```python
from build123d import *

# Parameters (mm, degrees)
SKETCH1_R           = 5.6
BOSS_EXTRUDE1_DEPTH = 3
SKETCH2_R           = 8.5
SKETCH2_R_2         = 5.6
BOSS_EXTRUDE2_DEPTH = 6
SKETCH3_R           = 8.5
BOSS_EXTRUDE3_DEPTH = 6
SKETCH4_R           = 1.6
CUT_EXTRUDE1_DEPTH  = 80.186488747
SKETCH5_R           = 3.3
CUT_EXTRUDE2_DEPTH  = 1.5
BOSS_EXTRUDE4_START = 6
SKETCH6_R           = 3.25
SKETCH6_R_2         = 1.6
BOSS_EXTRUDE4_DEPTH = 0.5


with BuildPart() as part:
    # Sketch1 → Boss-Extrude1 (new body)
    with BuildSketch(Plane.XY):
        with BuildLine():
            Line((6.873863542, 5), (63.126136458, 5))
            ThreePointArc((63.126136458, 5), (78.5, 0), (63.126136458, -5))
            Line((63.126136458, -5), (6.873863542, -5))
            ThreePointArc((6.873863542, -5), (-8.5, 0), (6.873863542, 5))
        make_face()
        Circle(SKETCH1_R, mode=Mode.SUBTRACT)
    extrude(amount=BOSS_EXTRUDE1_DEPTH)

    # Sketch2 → Boss-Extrude2 (add)
    with BuildSketch(Plane.XY):
        with Locations(Location((0, 0, 0), (0, 0, 323.968120928))):
            Circle(SKETCH2_R)
        Circle(SKETCH2_R_2, mode=Mode.SUBTRACT)
    extrude(amount=BOSS_EXTRUDE2_DEPTH)

    # Sketch3 → Boss-Extrude3 (add)
    with BuildSketch(Plane.XY):
        with Locations(Location((70, 0, 0), (0, 0, 216.031879072))):
            Circle(SKETCH3_R)
    extrude(amount=BOSS_EXTRUDE3_DEPTH)

    # Sketch4 → Cut-Extrude1 (cut, through all)
    with BuildSketch(Plane.XY):
        with Locations((70, 0)):
            Circle(SKETCH4_R)
    extrude(amount=CUT_EXTRUDE1_DEPTH, mode=Mode.SUBTRACT)

    # Sketch5 → Cut-Extrude2 (cut)
    with BuildSketch(Plane.XY):
        with Locations((70, 0)):
            Circle(SKETCH5_R)
    extrude(amount=CUT_EXTRUDE2_DEPTH, mode=Mode.SUBTRACT)

    # Sketch6 → Boss-Extrude4 (add)
    with BuildSketch(Plane.XY.offset(BOSS_EXTRUDE4_START)):
        with Locations((70, 0)):
            Circle(SKETCH6_R)
        with Locations((70, 0)):
            Circle(SKETCH6_R_2, mode=Mode.SUBTRACT)
    extrude(amount=BOSS_EXTRUDE4_DEPTH)


solid = part.part
```
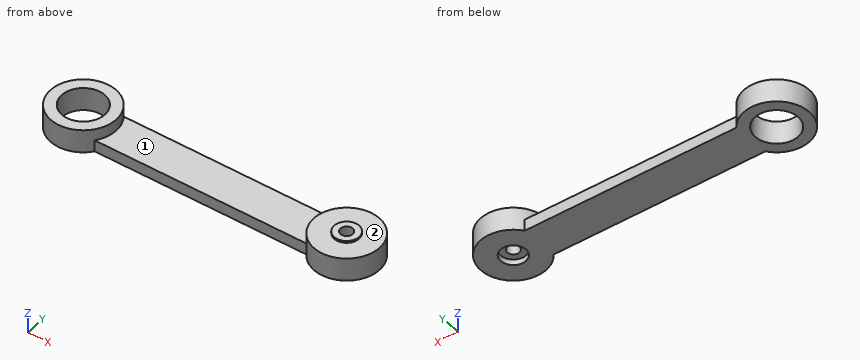
CAD build for the part. Positions are in the model's coordinates, mm. Face numbers are marked on the shaded views. Give positions to 0.01 mm unless a question says otherwise; leave off trailing zeros. Order: outer loops, then holes, each group sorted by start corner. A loop starts at its lowest first (then second) coordinate and runs counter-clockwise, first axis right, second up. Notation, with made-up numbers: M 58.25,-7 L 72.25,-7 A27 cw 72.25,30 Z; hole C 50,-7 d4. An arc over 180 degrees is marked long. Put each result on its own line as item: value. Start each with the question number.
(1) Mould opens along X. For the marked faces 1 and 2 say: +X half, -X half, draft (parallel to the pull), parting line (faces both ways), or undercut.
(2) Saw through at B-B, the plane y = 0. Write the cut outline in (x, z), then the cut area to 3 significant figures.
(3) Saw through at D-D, the plane x = 0. Write the cut outline in (y, z).
(4) Drill centre lines: line 1 along Y through (x, z) = (70, 1.15); line 2 along Y through (x, z) = (0, 2.6); line 3 along X through (y, z) = (-1.75, 3.75). Where is each one in solid material? Low to high.
(5) Flat gauge pins, fed straight in: pin 1 Ø0.9 at (x, z) = (22, 2) entering from -Y; pin 2 Ø0.9 at (x, z) = (29, 1.5) entering from +Y; pin 3 Ø2 at (x, y) = (71, -1) entering from -Z. Where does each tip first touch, or does it go through?
(6) Saw through at A-A, the plane x = 70. Write the cut outline in (y, z).
(7) Saw through at C-C, the plane z = 4.5. Write the cut outline in (x, y), then the cut area to 3 significant figures.
Check result:
1. face 1: undercut
1. face 2: draft
2. outline: M -8.5,0 L -5.6,0 L -5.6,6 L -8.5,6 Z; M 5.6,0 L 66.7,0 L 66.7,1.5 L 68.4,1.5 L 68.4,6.5 L 66.75,6.5 L 66.75,6 L 61.5,6 L 61.5,3 L 8.5,3 L 8.5,6 L 5.6,6 Z; M 71.6,1.5 L 73.3,1.5 L 73.3,0 L 78.5,0 L 78.5,6 L 73.25,6 L 73.25,6.5 L 71.6,6.5 Z
2. area: 273 mm2
3. outline: M -8.5,0 L -5.6,0 L -5.6,6 L -8.5,6 Z; M 5.6,0 L 8.5,0 L 8.5,6 L 5.6,6 Z
4. line 1: y = -8.5 to -3.3, 3.3 to 8.5
4. line 2: y = -8.5 to -5.6, 5.6 to 8.5
4. line 3: x = -8.32 to -5.32, 5.32 to 8.32, 61.68 to 78.32
5. pin 1: stops at y = -5
5. pin 2: stops at y = 5
5. pin 3: stops at z = 1.5
6. outline: M -8.5,0 L -3.3,0 L -3.3,1.5 L -1.6,1.5 L -1.6,6.5 L -3.25,6.5 L -3.25,6 L -8.5,6 Z; M 1.6,1.5 L 3.3,1.5 L 3.3,0 L 8.5,0 L 8.5,6 L 3.25,6 L 3.25,6.5 L 1.6,6.5 Z
7. outline: C 0,0 d17; C 70,0 d17; hole C 0,0 d11.2; hole C 70,0 d3.2
7. area: 347 mm2
